Build history of the part. All positions in model axes, mm. Round coordinates to 2 decimals unless told otherwise and drop trailing zeros. Write each loop counter-clockwise with the first axis right and the second up, starting at its lowest first coordinate (ties: lowest second). Pieces come first, ordered by that corner, then holes. Notation, with made-up numbers: (41.25, 18) -> (88.25, 18) arc R20 cw to (88.25, 49) -> close; hole circle Ø10 at (65, -29.75). An arc over 180 degrees is marked (long way). Return JSON: item names as keys, results as strings.
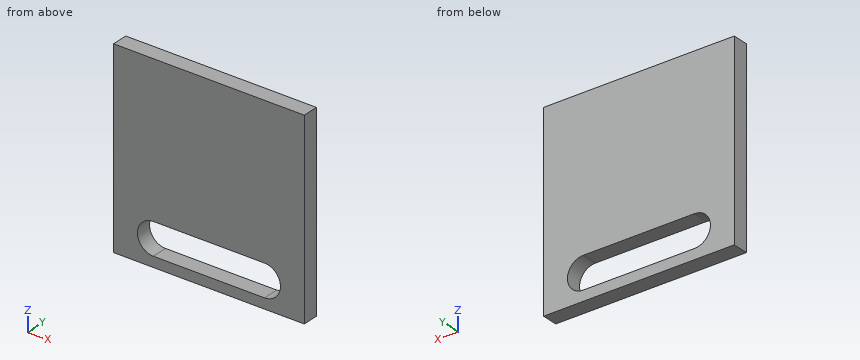
from build123d import *

# Parameters (mm, degrees)
F0_W     = 76.2
F0_H     = 76.2
F1_DEPTH = 3.175
F2_W     = 44.45
F2_H     = 12.7
F3_DEPTH = 6.35


with BuildPart() as f1:
    # F0 (on Front) → F1 (new body, symmetric)
    with BuildSketch(Plane.XZ):
        with Locations((0, 38.1)):
            Rectangle(F0_W, F0_H)
    extrude(amount=F1_DEPTH, both=True)

    # F2 (on face) → F3 (cut)
    with BuildSketch(Plane.XZ.offset(3.175)):
        with BuildLine():
            Line((-22.225, 4.1064423469), (-22.225, 16.8064423469))
            ThreePointArc((-22.225, 16.8064423469), (-28.575, 10.4564423469), (-22.225, 4.1064423469))
        make_face()
        with Locations((0, 10.4564423469)):
            Rectangle(F2_W, F2_H)
        with BuildLine():
            ThreePointArc((22.225, 4.1064423469), (28.575, 10.4564423469), (22.225, 16.8064423469))
            Line((22.225, 16.8064423469), (22.225, 4.1064423469))
        make_face()
    extrude(amount=-F3_DEPTH, mode=Mode.SUBTRACT)


solid = f1.part
Q1. Saw through at C-C on x = 25.5. List the corners of the cut face in (y, z) (3 decimals), then the cut area to 3 significant figures.
Verdict:
{"outline": "(-3.175, 0) -> (3.175, 0) -> (3.175, 5.016) -> (-3.175, 5.016) -> close; (-3.175, 15.897) -> (3.175, 15.897) -> (3.175, 76.2) -> (-3.175, 76.2) -> close", "area": "415 mm²"}
Q2. Wall check: L1, parallel to Z at x = -2, y = 0.75; L2, parallel to X at y = 1, z = 13.5. Give the ranges that are in metal, low to high.
Verdict:
{"L1": "z = 0 to 4.11, 16.81 to 76.2", "L2": "x = -38.1 to -27.8, 27.8 to 38.1"}
Q3. Saw through at B-B on y = -1.25. List the corners of the cut face in (x, z) (3 decimals), then the cut area to 3 significant figures.
Verdict:
{"outline": "(-38.1, 0) -> (38.1, 0) -> (38.1, 76.2) -> (-38.1, 76.2) -> close; hole (-22.225, 4.106) -> (22.225, 4.106) arc R6.35 ccw to (22.225, 16.806) -> (-22.225, 16.806) arc R6.35 ccw to start", "area": "5,120 mm²"}
Q4. Saw through at A-A on x = -4. List the corners of the cut face in (y, z) (3 decimals).
Verdict:
{"outline": "(-3.175, 0) -> (3.175, 0) -> (3.175, 4.106) -> (-3.175, 4.106) -> close; (-3.175, 16.806) -> (3.175, 16.806) -> (3.175, 76.2) -> (-3.175, 76.2) -> close"}
